Study the drawing (mm; zero at the part's minimum x, y, z) and answer. Coordinates: 2 decimals unless noted, no trailing zeros. Loops run counter-clockwise (first coordinate to the right, second up) from the corner with the lowest first, then second, coordinate; pieces in that order, holes last. Notation, with made-up numbers: (60.5, -14) -> (107.5, -14) arc R27 cw to (107.5, 6) -> close; hole circle Ø3 at (32.5, -29). An arc over 180 degrees is marked (long way). Answer in a Markdown table with one row per item.
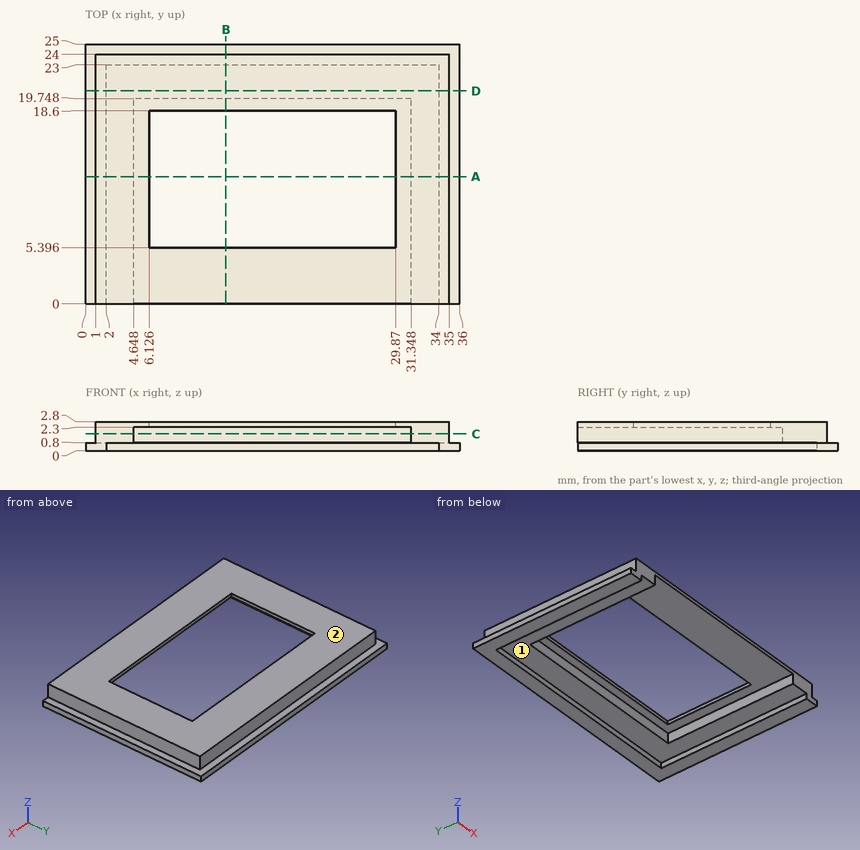
1. Given pin 1 Ø1.2 at (y, z) = (10.5, 1.5) entering from -X; pin 2 Ø0.6 at (x, z) = (20, 1.5) entering from +Y; pin 3 Ø0.6 at (y, z) = (6.5, 1.5) entering from +X, each flat-ended and moving along its own axis, determine where each tip first touches the part or whether it passes through.
A:
| item | result |
|---|---|
| pin 1 | stops at x = 1 |
| pin 2 | stops at y = 24 |
| pin 3 | stops at x = 35 |
2. A cutting plane is placed at B-B on x = 13.5. Give the vertices of the cut face in (y, z), and give its area (3 significant figures).
A:
| item | result |
|---|---|
| outline | (0, 2.3) -> (5.4, 2.3) -> (5.4, 2.8) -> (0, 2.8) -> close; (18.6, 2.3) -> (19.75, 2.3) -> (19.75, 0.8) -> (23, 0.8) -> (23, 0) -> (25, 0) -> (25, 0.8) -> (24, 0.8) -> (24, 2.8) -> (18.6, 2.8) -> close |
| area | 13.4 mm2 |
3. A cutting plane is placed at C-C on z = 1.65. Give the vertices of the cut face in (x, y), and give its area (3 significant figures).
A:
| item | result |
|---|---|
| outline | (1, 0) -> (4.65, 0) -> (4.65, 19.75) -> (31.35, 19.75) -> (31.35, 0) -> (35, 0) -> (35, 24) -> (1, 24) -> close |
| area | 289 mm2 |
4. Find the intervals of material crossed by probe 1 along X at (y, z) = (19.25, 1.9); probe 2 along X at (y, z) = (6, 0.2); probe 3 along Y at (x, z) = (5.5, 2.6), in increasing order.
A:
| item | result |
|---|---|
| probe 1 | x = 1 to 4.65, 31.35 to 35 |
| probe 2 | x = 0 to 2, 34 to 36 |
| probe 3 | y = 0 to 24 |
5. A cutting plane is placed at A-A on y = 12.25. Give the vertices of the cut face in (x, z).
A:
| item | result |
|---|---|
| outline | (0, 0) -> (2, 0) -> (2, 0.8) -> (4.65, 0.8) -> (4.65, 2.3) -> (6.13, 2.3) -> (6.13, 2.8) -> (1, 2.8) -> (1, 0.8) -> (0, 0.8) -> close; (29.87, 2.3) -> (31.35, 2.3) -> (31.35, 0.8) -> (34, 0.8) -> (34, 0) -> (36, 0) -> (36, 0.8) -> (35, 0.8) -> (35, 2.8) -> (29.87, 2.8) -> close |
6. The mould has two halves that part along X. Classify the marked faces 1 and 2: pulls with the +X half, pulls with the -X half, needs draft (parallel to the pull), parting line crosses it, or undercut.
A:
| item | result |
|---|---|
| face 1 | undercut |
| face 2 | needs draft |
7. A cutting plane is placed at D-D on y = 20.5. Give the vertices of the cut face in (x, z), and give its area (3 significant figures).
A:
| item | result |
|---|---|
| outline | (0, 0) -> (2, 0) -> (2, 0.8) -> (34, 0.8) -> (34, 0) -> (36, 0) -> (36, 0.8) -> (35, 0.8) -> (35, 2.8) -> (1, 2.8) -> (1, 0.8) -> (0, 0.8) -> close |
| area | 71.2 mm2 |
